Could you check a few things on this model? Use its own coordinates, in mm. A direction names the side the tool comes from. Coordinates: 2 decimals unless noted, no trailing zeros. Write each loop counter-clockwise with the first axis right and the second up, starting at its lowest first coordinate (ties: lowest second). Pieces come first, ordered by that corner, then holes. Notation, with made-up numbers: (23.25, 56.5) - (58.25, 56.5) arc R27 cw to (58.25, 93.5) - close; hole circle Ø4 at (77, 6). An arc over 180 degrees is marked (long way). Write item = value, one per line. Start each with the question number.
Autodesk Inventor part; units mm, degrees
ref_plane "YZ Plane" through (0, 0, 0) normal (1, 0, 0) x (0, 1, 0)
ref_plane "XZ Plane" through (0, 0, 0) normal (0, 1, 0) x (-1, 0, 0)
ref_plane "XY Plane" through (0, 0, 0) normal (0, 0, 1) x (1, 0, 0)
sketch "Sketch1" plane through (0, 0, 0) normal (0, 0, 1) x (1, 0, 0)
  line L0 (-262.5, 0) -> (262.5, 0) construction
  line L1 (0, -52.5) -> (0, 52.5) construction
  line L2 (-187.5, 37.5) -> (187.5, 37.5)
  line L3 (187.5, 37.5) -> (187.5, -37.5)
  line L4 (187.5, -37.5) -> (-187.5, -37.5)
  line L5 (-187.5, -37.5) -> (-187.5, 37.5)
  point P0 (-175, 25)
  point P1 (175, 25)
  point P2 (-175, -25)
  point P3 (175, -25)
  point P4 (0, 0)
  point P5 (-175, 0)
  point P6 (175, 0)
  point P7 (0, 25)
  point P8 (0, -25)
  dimension "d0" = 375
  dimension "d1" = 75
  dimension "d3" = 350
  dimension "d30" = 12.5
  dimension "d45" = 12.5
extrude "Extrusion1" add sketch "Sketch1" against normal blind 10
hole "Hole1" at (-175, 25, 0) at (175, 25, 0) at (-175, -25, 0) at (175, -25, 0) at (0, 25, 0) at (0, -25, 0) direction (0, 0, -1) diameter 6.6 end through all countersink diameter 14.5 countersink angle 90
hole "Hole2" at (0, 0, 0) direction (0, 0, -1) diameter 10.647 end through all
hole "Hole3" at (-175, 0, 0) at (175, 0, 0) direction (0, 0, -1) diameter 20 depth 1
sketch "Sketch2" plane through (0, 0, -10) normal (0, 0, -1) x (-1, 0, 0)
  circle A0 centre (175, 0) radius 10
  circle A1 centre (-175, 0) radius 10
  point P0 (0, 0)
hole "Hole4" at (-175, 0, -10) at (175, 0, -10) direction (0, 0, 1) diameter 6.6 end through all countersink diameter 14.5 countersink angle 90
chamfer "Chamfer1" distance 2 angle 45 4 edges at (-187.5, 37.5, -5) (-187.5, -37.5, -5) (187.5, 37.5, -5) (187.5, -37.5, -5)
properties part number "DLT-01-235B" material "Aluminio 1060"
1) Suppose I cut it at D-D on y = 25. Please give me the cut outline in (x, z), plus the area to 3 significant figures.
2) If I drill on probe 1 along X at (y, z) = (-25, -5.25); probe 2 along X at (y, z) = (0, -3.9); probe 3 along Y at (x, z) = (175, -6), over which ranges is the centre line in solid material (lowest first)? Write a range as [from, to].
3) For P1, Ø8.5, axis at x = -175, y = 25, coming from the +Z side; P2, Ø10, axis at x = 177, y = 4.5, coming from the +Z side; P3, Ø10.5, axis at x = 175, y = 0, coming from the -Z side; P4, Ø5, axis at x = 130, y = 8, coming from the +Z side, each with a flat end and sliding along its axis, tell me the tip position at first contact or that it passes through.
4) Suppose I cut it at A-A on y = 0. Please give me the cut outline in (x, z).
5) Suppose I cut it at C-C on z = -8. State how many separate pieces and enclosed holes the cut face has, plus the area to 3 significant figures.
6) Which directions (+Z, -Z, +X, -X, +Y, -Y) give clear straight access to the entire face, cutting with the end or side of a thin tool? Please do faces 1 (the flat face through (-175, -4, -1)), 2 (the cylindrical face through (1.26, 21.95, -7.02)).
7) Suppose I cut it at B-B on x = 175. Please give me the cut outline in (y, z).
8) Thinking about a two-plate mould opening in X: for faces 3 (the cylindrical face through (178.22, -0.72, -3.49)), 4 (the flat face through (-3, 9, -10)), which applies, +X half, -X half, draft (parallel to the pull), parting line (faces both ways), or undercut?
Reply:
q1.outline = (-187.5, -10) - (-178.3, -10) - (-178.3, -3.95) - (-182.25, 0) - (-187.5, 0) - close; (-171.7, -10) - (-3.3, -10) - (-3.3, -3.95) - (-7.25, 0) - (-167.75, 0) - (-171.7, -3.95) - close; (3.3, -10) - (171.7, -10) - (171.7, -3.95) - (167.75, 0) - (7.25, 0) - (3.3, -3.95) - close; (178.3, -10) - (187.5, -10) - (187.5, 0) - (182.25, 0) - (178.3, -3.95) - close
q1.area = 3,510 mm^2
q2.probe_1 = [-187.5, -178.3], [-171.7, -3.3], [3.3, 171.7], [178.3, 187.5]
q2.probe_2 = [-187.5, -178.3], [-171.7, -5.32], [5.32, 171.7], [178.3, 187.5]
q2.probe_3 = [-37.5, -28.3], [-21.7, -3.3], [3.3, 21.7], [28.3, 37.5]
q3.P1 = -3
q3.P2 = -1
q3.P3 = -8
q3.P4 = 0
q4.outline = (-187.5, -10) - (-182.25, -10) - (-178.3, -6.05) - (-178.3, -1) - (-185, -1) - (-185, 0) - (-187.5, 0) - close; (-171.7, -6.05) - (-167.75, -10) - (-5.32, -10) - (-5.32, 0) - (-165, 0) - (-165, -1) - (-171.7, -1) - close; (5.32, -10) - (167.75, -10) - (171.7, -6.05) - (171.7, -1) - (165, -1) - (165, 0) - (5.32, 0) - close; (178.3, -6.05) - (182.25, -10) - (187.5, -10) - (187.5, 0) - (185, 0) - (185, -1) - (178.3, -1) - close
q5.separate_pieces = 1
q5.enclosed_holes = 9
q5.area = 27,600 mm^2
q6.face_1 = +Z
q6.face_2 = +Z, -Z
q7.outline = (-37.5, -10) - (-28.3, -10) - (-28.3, -3.95) - (-32.25, 0) - (-37.5, 0) - close; (-21.7, -10) - (-7.25, -10) - (-3.3, -6.05) - (-3.3, -1) - (-10, -1) - (-10, 0) - (-17.75, 0) - (-21.7, -3.95) - close; (3.3, -6.05) - (7.25, -10) - (21.7, -10) - (21.7, -3.95) - (17.75, 0) - (10, 0) - (10, -1) - (3.3, -1) - close; (28.3, -10) - (37.5, -10) - (37.5, 0) - (32.25, 0) - (28.3, -3.95) - close
q8.face_3 = undercut
q8.face_4 = draft
